Input: dimensioned drawing with shaded views. Units: mm. Origin: part minimum x, y, z. A direction names the side the tool comes from. Round coordinates to 2 decimals unless told otherwise and drop trailing zeros. Loops run counter-clockwise (first coordinate to the right, second up) from the corner with the lowest first, then second, coordinate; pieces in that order, holes last. Notation, with made-up numbers: (14, -10.75) - (45, -10.75) arc R7 ccw to (45, -5.75) - close; hole circle Ø6 at (-27, -3). An arc over 180 degrees is marked (long way). Answer as a JSON object with one key per item and string values. Group by question number.
Item 1: Line query: line 1 (X direction, y = 6, z = 12); line 2 (Z direction, x = 50, y = 6); line 3 (Z direction, x = 31.5, y = 29). Output: solid intervals per line, ascending.
Item 2: Section A-A (z = 11). Return the cut outline in (x, y).
Item 3: Reachability of the marked faces 4, 5 and 6 from +Z, -Z, +X, -X, +Y, -Y: full face, straight path, thin tool, end or side. Return the list, or none.
Item 4: Draft query along Y for the marked faces 1, 2 and 3. Return one class per face: released by +Y, released by -Y, zero draft, split by the parting line, or undercut.
Item 5: First-contact query: pin 1 (10.5 mm diameter, centred on x = 62, z = 27.5, fed in from +Y); pin 2 (10 mm diameter, centred on x = 55, y = 29.5, fed in from -Z); pin 3 (5 mm diameter, centred on x = 54.5, z = 19, fed in from -Y); pin 4 (4 mm diameter, centred on y = 39, z = 23.5, fed in from -X). Flat tips, straight axial feed; report the tip coordinate or a pass-through.
Item 6: Section C-C (z = 26.5). Return the cut outline in (x, y), plus the area to 3 significant figures.
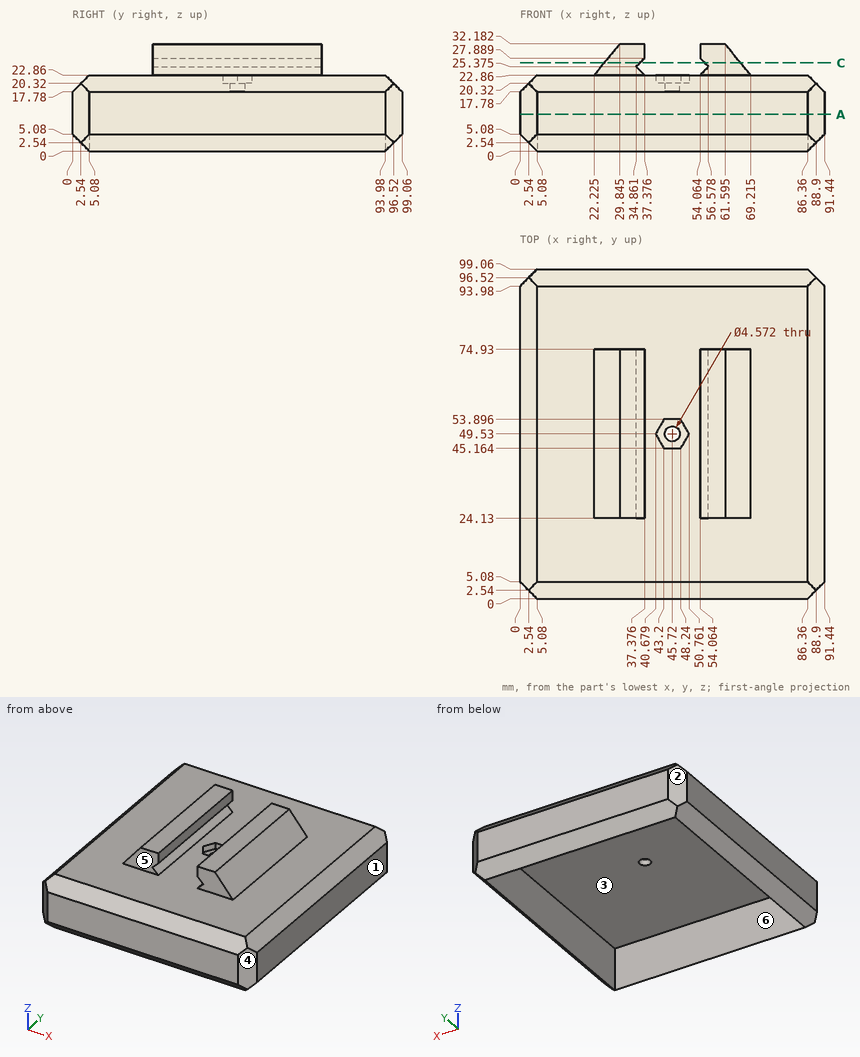
Values:
{
 "1": {"line 1": "x = 0 to 5.08, 86.36 to 91.44", "line 2": "z = 17.78 to 22.86", "line 3": "z = 17.78 to 32.18"},
 "2": {"outline": "(0, 5.08) - (5.08, 0) - (86.36, 0) - (91.44, 5.08) - (91.44, 93.98) - (86.36, 99.06) - (5.08, 99.06) - (0, 93.98) - close; hole (5.08, 5.08) - (86.36, 5.08) - (86.36, 93.98) - (5.08, 93.98) - close"},
 "3": {"face 4": "+Z, -Z, +X, -Y", "face 5": "+Z, +X, -X, -Y", "face 6": "-Z"},
 "4": {"face 1": "zero draft", "face 2": "released by +Y", "face 3": "undercut"},
 "5": {"pin 1": "stops at y = 94.59", "pin 2": "stops at z = 17.78", "pin 3": "stops at y = 0", "pin 4": "stops at x = 3.72"},
 "6": {"outline": "(25.2, 24.13) - (35.99, 24.13) - (35.99, 74.93) - (25.2, 74.93) - close; (55.45, 24.13) - (66.24, 24.13) - (66.24, 74.93) - (55.45, 74.93) - close", "area": "1,100 mm^2"}
}
